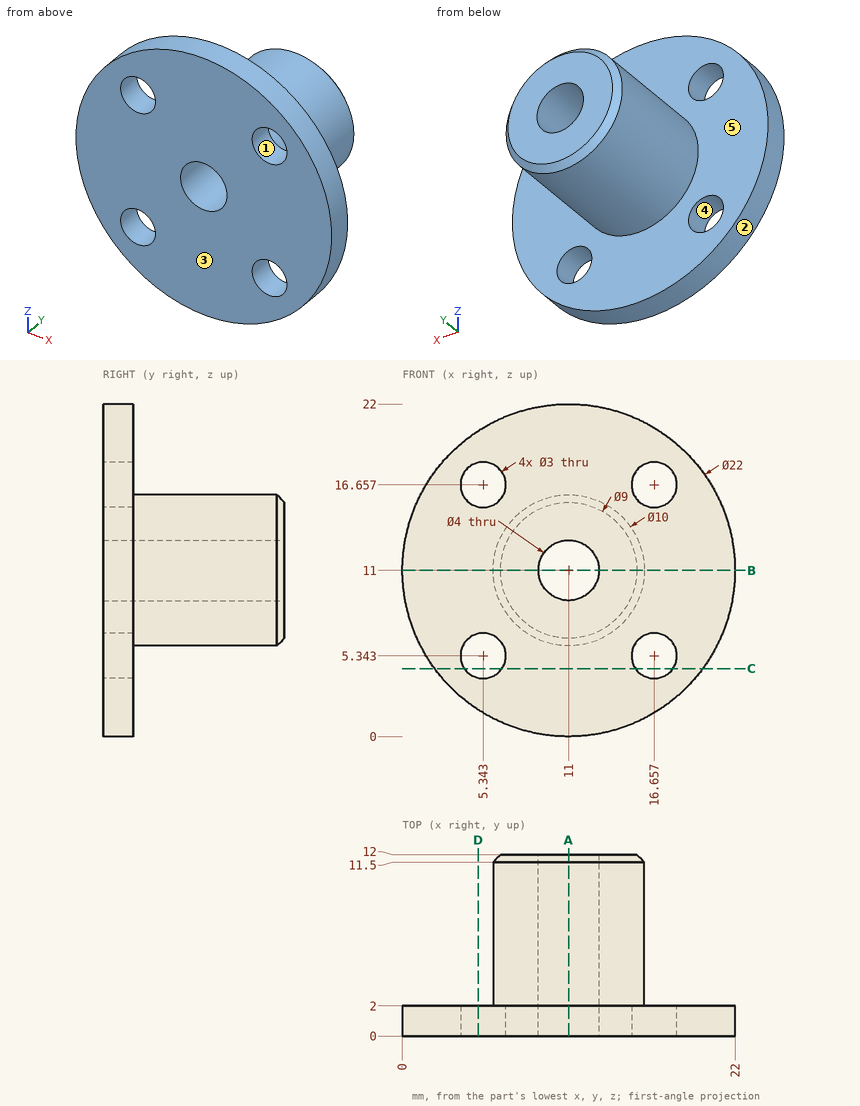
For this review, use the dimensioned drawing (mm, ordinates from the lowest corner) and the shaded views. A direction names the side the tool comes from. Round coordinates to 2 decimals unless told otherwise and drop trailing zeros. Write each loop counter-clockwise with the first axis right and the second up, starting at its lowest first coordinate (ties: lowest second). Pieces come first, ordered by that corner, then holes. Notation, with made-up numbers: (49, 10.5) - (61, 10.5) arc R8 cw to (61, 18.5) - close; hole circle Ø8 at (18, 88). An arc over 180 degrees is marked (long way). Answer as CSV lines item,"result". Start each with the question number.
(1) Draft analysis for pull direction X (two halves, no side actions). For the marked faces 1, 2 and 3, state which applies: pulls with the +X half, pulls with the -X half, needs draft (parallel to the pull), parting line crosses it, or undercut.
(2) We need section D-D on x = 5. State the section outline as (y, z) points.
(3) For pin 1 Ø5 at (y, z) = (10, 5.5) entering from +X; pin 2 Ø2.5 at (x, z) = (16.66, 16.66) entering from +Y; pin 3 Ø3 at (x, y) = (11, 6.5) entering from -Z; pin 4 Ø1 at (x, y) = (7, 4.5) entering from -Z, all flat-tipped, find the tip position at first contact; note any pin that passes through.
(4) We need section A-A on x = 11. State the section outline as (y, z) points.
(5) To check wall thickness, follow line 1 (X direction, y = 4, z = 11); line 2 (Y direction, x = 9.25, z = 2.25). State the ranges of each line that lie inside material, in increasing order.
(6) We need section B-B on z = 11. State the section outline as (x, y) points.
(7) We need section C-C on z = 4.5. State the section outline as (x, y) points, plus the area to 3 significant figures.
(8) For the marked faces 4 and 5, list the 3-axis set-ups (+Z, -Z, +X, -X, +Y, -Y) from which the entire face can be reached by the end or side of a thin tool; tool diameter is ignored.
Worked answers:
1,face 1,"undercut"
1,face 2,"parting line crosses it"
1,face 3,"needs draft"
2,outline,"(0, 1.78) - (2, 1.78) - (2, 3.88) - (0, 3.88) - close; (0, 6.8) - (2, 6.8) - (2, 15.2) - (0, 15.2) - close; (0, 18.12) - (2, 18.12) - (2, 20.22) - (0, 20.22) - close"
3,pin 1,"x = 15"
3,pin 2,"through"
3,pin 3,"z = 6"
3,pin 4,"z = 7.43"
4,outline,"(0, 0) - (2, 0) - (2, 6) - (11.5, 6) - (12, 6.5) - (12, 9) - (0, 9) - close; (0, 13) - (12, 13) - (12, 15.5) - (11.5, 16) - (2, 16) - (2, 22) - (0, 22) - close"
5,line 1,"6 to 9, 13 to 16"
5,line 2,"0 to 2"
6,outline,"(0, 0) - (9, 0) - (9, 12) - (6.5, 12) - (6, 11.5) - (6, 2) - (0, 2) - close; (13, 0) - (22, 0) - (22, 2) - (16, 2) - (16, 11.5) - (15.5, 12) - (13, 12) - close"
7,outline,"(2.13, 0) - (4.1, 0) - (4.1, 2) - (2.13, 2) - close; (6.58, 0) - (15.42, 0) - (15.42, 2) - (6.58, 2) - close; (17.9, 0) - (19.87, 0) - (19.87, 2) - (17.9, 2) - close"
7,area,"25.6 mm²"
8,face 4,"+Y, -Y"
8,face 5,"+Y"
